```python
from build123d import *

# Parameters (mm, degrees)
F1_DEPTH    = 12.7
F2_R        = 5.08
F3_T1_DEPTH = 255.9982991577
F3_T3_DEPTH = 445.2282991577
F3_T5_DEPTH = 375.3782991577


# Not quite as in the source:
# - a fillet or chamfer that OpenCascade refuses, or shapes differently, is made with other operations: its cross-section is extruded or revolved along the edge and cut away or added


with BuildPart() as f1:
    # F0 (on Front) → F1 (new body)
    with BuildSketch(Plane.XZ):
        with BuildLine():
            Line((55.5559131622, 244.2450298561), (-179.3940868378, 244.2450298561))
            Line((-179.3940868378, 244.2450298561), (-179.3940868378, -174.8549701439))
            Line((-179.3940868378, -174.8549701439), (169.8559131622, -174.8549701439))
            Line((169.8559131622, -174.8549701439), (169.8559131622, 231.5450298561))
            Line((169.8559131622, 231.5450298561), (68.2559131622, 231.5450298561))
            ThreePointArc((68.2559131622, 231.5450298561), (59.2756570412, 235.264773735), (55.5559131622, 244.2450298561))
        make_face()
    extrude(amount=F1_DEPTH)

    # F2
    f2_edges = [f1.edges().sort_by_distance(p)[0] for p in [
        (119.055913, 0, 231.54503),
        (119.055913, -12.7, 231.54503),
        (59.275657, 0, 235.264774),
        (59.275657, -12.7, 235.264774),
    ]]
    fillet(f2_edges, radius=F2_R)

    # F3: chamfer of 5.08 on 3 edges, made by hand

    # F3_s2 → F3_t1 (cut)
    with BuildSketch(Plane.YZ.offset(-192.4582364166)):
        Polygon((-5.08, 244.2450298561), (0, 239.1650298561), (0, 244.2450298561), align=None)
    extrude(amount=F3_T1_DEPTH, mode=Mode.SUBTRACT)

    # F3_s4 → F3_t3 (cut)
    with BuildSketch(Plane.XY.offset(-187.9191197228)):
        Polygon((-174.3140868378, 0), (-179.3940868378, -5.08), (-179.3940868378, 0), align=None)
    extrude(amount=F3_T3_DEPTH, mode=Mode.SUBTRACT)

    # F3_s6 → F3_t5 (cut)
    with BuildSketch(Plane.YZ.offset(-192.4582364166)):
        Polygon((0, -169.7749701439), (-5.08, -174.8549701439), (0, -174.8549701439), align=None)
    extrude(amount=F3_T5_DEPTH, mode=Mode.SUBTRACT)


solid = f1.part
```
Input: part model. Units: mm. Frame: model coordinates. Give positions to 0.01 mm unless a question says otherwise; leave off trailing zeros. Order: outer loops, then holes, each group sorted by start corner. A loop starts at its lowest first (then second) coordinate and runs counter-clockwise, first axis right, second up. Notation, with made-up numbers: M 30.25,20 L 62.25,20 A23 cw 62.25,37 Z; hole C 19,69.25 d2. An arc over 180 degrees is marked long. One line per question, with ' | ' between items.
1) Contact query for flat-ended pins moving along their axis: P1, Ø0.8, axis at x = 125.5, y = -6.5, coming from the +Z side (3 decimals); P2, Ø1, axis at x = 43, y = -2, coming from the +Z side (3 decimals); P3, Ø1, axis at x = -106, y = -4, coming from the -Z side (3 decimals). Output: stop coordinate, or through.
Filled in:
P1: stops at z = 231.545 | P2: stops at z = 241.665 | P3: stops at z = -174.275
2) Section A-A on y = -2. Output: boundary loops of the cut face in (x, z), and give its area (3 significant figures).
Filled in:
outline: M -176.31,-171.77 L 169.86,-171.77 L 169.86,230.5 L 68.26,230.5 A13.74 cw 54.87,241.17 L -176.31,241.17 Z | area: 142,000 mm2
3) Ray query, L1, parallel to Z at x = 155, y = -6.75; L2, parallel to X at y = -3, z = -44.5; L3, parallel to Z at x = 83, y = -4. Return the intervals inside material, ascending.
Filled in:
L1: z = -174.85 to 231.55 | L2: x = -177.31 to 169.86 | L3: z = -173.77 to 231.43
